Work out the finished part from the listing and answer in its coordinate system (mm). A direction names the side the tool comes from. Coordinates: 2 decimals unless noted, no trailing zeros. Order: outer loops, then holes, each group sorted by start corner. A loop starts at its lowest first (then second) coordinate and runs counter-clockwise, first axis right, second up. Notation, with made-up numbers: M 85.5,72 L 144.5,72 A19 cw 144.5,94 Z; hole C 33,34 d7. An arc over 180 degrees is marked long. Use a Markdown table: item, result. Add a question column.
from build123d import *

# Parameters (mm, degrees)
SKETCH1_W           = 40
SKETCH1_H           = 30
BOSS_EXTRUDE1_DEPTH = 6
SKETCH2_R           = 1.5
CUT_EXTRUDE1_DEPTH  = 6
FILLET1_R           = 4
SKETCH3_W           = 21
SKETCH3_H           = 21
CUT_EXTRUDE2_DEPTH  = 4


with BuildPart() as part:
    # Sketch1 → Boss-Extrude1 (new body)
    with BuildSketch(Plane(origin=(0, 0, 0), x_dir=(1, 0, 0), z_dir=(0, 1, 0))):
        with Locations((20, 15)):
            Rectangle(SKETCH1_W, SKETCH1_H)
    extrude(amount=BOSS_EXTRUDE1_DEPTH)

    # Sketch2 → Cut-Extrude1 (cut)
    with BuildSketch(Plane(origin=(0, 6, 0), x_dir=(1, 0, 0), z_dir=(0, 1, 0))):
        with Locations(Location((5, 5, 0), (0, 0, 270))):
            Circle(SKETCH2_R)
        with Locations(Location((5, 25, 0), (0, 0, 90))):
            Circle(SKETCH2_R)
        with Locations(Location((35, 5, 0), (0, 0, 90))):
            Circle(SKETCH2_R)
        with Locations(Location((35, 25, 0), (0, 0, 270))):
            Circle(SKETCH2_R)
    extrude(amount=-CUT_EXTRUDE1_DEPTH, mode=Mode.SUBTRACT)

    # Fillet1
    fillet1_edges = [part.edges().sort_by_distance(p)[0] for p in [
        (0, 3, -30),
        (40, 3, -30),
        (40, 3, 0),
        (0, 3, 0),
    ]]
    fillet(fillet1_edges, radius=FILLET1_R)

    # Sketch3 → Cut-Extrude2 (cut)
    with BuildSketch(Plane(origin=(0, 6, 0), x_dir=(1, 0, 0), z_dir=(0, 1, 0))):
        with Locations((20, 15)):
            Rectangle(SKETCH3_W, SKETCH3_H)
    extrude(amount=-CUT_EXTRUDE2_DEPTH, mode=Mode.SUBTRACT)


solid = part.part
(1) A cutting plane is placed at C-C on y = 0.6. Write down the section's boundary in (x, z), plus the area to 3 significant figures.
(2) Given P1, Ø4, axis at x = 18.5, z = -9.5, coming from the +Y side, flat-ended and moving along its own axis, determine where the tip first touches the part or whether it passes through.
(3) A cutting plane is placed at B-B on x = 5. Write down the section's boundary in (y, z).
(4) A cutting plane is placed at D-D on x = 23.5. Write down the section's boundary in (y, z), plus the area to 3 significant figures.
(5) The mould has two halves that part along X. Classify faces 3 (the cylindrical face through (38.797, 3.042, -28.859)), 4 (the flat face through (9.5, 4, -15)), 5 (the cylindrical face through (1.141, 3.042, -1.203)), 6 (the flat face through (30.5, 4, -15)): pulls with the +X half, pulls with the -X half, needs draft (parallel to the pull), parting line crosses it, or undercut.
(6) Straight lines are drawn through the part: line 1 (X direction, y = 2.4, z = -5); line 2 (Z direction, x = 27, y = 5.2); line 3 (X direction, y = 0.75, z = -24). For each, find the intervals that lie inside material, in ascending order.
(7) A cutting plane is placed at A-A on z = -5. Write down the section's boundary in (x, y).
(8) Which of the six approach directions +Z, -Z, +X, -X, +Y, -Y give full straight-line access (tool end or side, diameter ignored) to faces 1 (the cylindrical face through (38.797, 3.042, -1.141)), 2 (the flat face through (20, 4, -25.5))?
From the geometry:
| question | item | result |
|---|---|---|
| 1 | outline | M 0,-26 A4 ccw 4,-30 L 36,-30 A4 ccw 40,-26 L 40,-4 A4 ccw 36,0 L 4,0 A4 ccw 0,-4 Z; hole C 5,-25 d3; hole C 5,-5 d3; hole C 35,-25 d3; hole C 35,-5 d3 |
| 1 | area | 1,160 mm2 |
| 2 | P1 | stops at y = 2 |
| 3 | outline | M 0,-30 L 6,-30 L 6,-26.5 L 0,-26.5 Z; M 0,-23.5 L 6,-23.5 L 6,-6.5 L 0,-6.5 Z; M 0,-3.5 L 6,-3.5 L 6,0 L 0,0 Z |
| 4 | outline | M 0,-30 L 6,-30 L 6,-25.5 L 2,-25.5 L 2,-4.5 L 6,-4.5 L 6,0 L 0,0 Z |
| 4 | area | 96.0 mm2 |
| 5 | face 3 | pulls with the +X half |
| 5 | face 4 | undercut |
| 5 | face 5 | pulls with the -X half |
| 5 | face 6 | undercut |
| 6 | line 1 | x = 0 to 3.5, 6.5 to 9.5, 30.5 to 33.5, 36.5 to 40 |
| 6 | line 2 | z = -30 to -25.5, -4.5 to 0 |
| 6 | line 3 | x = 0 to 3.88, 6.12 to 33.88, 36.12 to 40 |
| 7 | outline | M 0,0 L 3.5,0 L 3.5,6 L 0,6 Z; M 6.5,0 L 33.5,0 L 33.5,6 L 30.5,6 L 30.5,2 L 9.5,2 L 9.5,6 L 6.5,6 Z; M 36.5,0 L 40,0 L 40,6 L 36.5,6 Z |
| 8 | face 1 | +Z, +X, +Y, -Y |
| 8 | face 2 | +Y |
